For this review, take the finished solid that the model builds, in its own axes (mm). A direction names the side the tool comes from. Give positions to 0.01 mm unless a question says otherwise; leave off trailing zeros. Order: outer loops, then holes, each group sorted by start corner. A loop starts at its lowest first (then second) coordinate and runs counter-clockwise, first axis right, second up.
Item 1: For P1, Ø2, axis at x = -14.5, z = 5, coming from the -Y side; P2, Ø3, axis at x = -7, z = 9.5, coming from the -Y side; P3, Ø8, axis at x = -13.5, y = 2.5, coming from the +Z side, all flat-tipped, find the tip position at first contact; note any pin that passes through.
Item 2: Consider section D-D (y = 12). Give the boundary of the cut face in (x, z).
Item 3: For probe 1 along Z at (x, y) = (-6, -18); probe 2 along X at (y, z) = (-2, 17.25); probe 3 along X at (y, z) = (-0.5, 12.5), list the stretches that pass through material, from the lowest coordinate up.
Item 4: Machinability: for faces 1 (the cylindrical face through (-4.336, -19.524, 4.93)), 2 (the flat face through (4, -4, 10)), 3 (the cylindrical face through (0, -2, 2)), which of the approach directions +Z, -Z, +X, -X, +Y, -Y give a long, thin tool a straight path to every point of the face, cutting with its end or side? Answer none if there is none.
Item 5: Consider section B-B (x = 0). Give the boundary of the cut face in (y, z), plus the area to 3 significant figures.
Item 6: Consider section C-C (z = 6.5). Give the boundary of the cut face in (x, y), plus the area to 3 significant figures.
Item 7: The part is to be moulded in two halves that separate along Y. For faces 4 (the cylindrical face through (-1.08, -4.88, 16.41)), 5 (the flat face through (0, 0, 23)), 6 (the flat face through (0, 0, 5)), say which applies: released by +Y, released by -Y, zero draft, split by the parting line, or undercut.
Item 8: Consider section A-A (y = 0). Give the boundary of the cut face in (x, z), plus the area to 3 significant figures.
```python
from build123d import *

# Parameters (mm, degrees)
F0_R     = 20
F1_DEPTH = 10
F2_R     = 5
F3_DEPTH = 13
F5_DEPTH = 5


with BuildPart() as f1:
    # F0 (on Top) → F1 (new body)
    with BuildSketch(Plane.XY):
        Circle(F0_R)
    extrude(amount=F1_DEPTH)

    # F2 (on face) → F3 (join)
    with BuildSketch(Plane.XY.offset(10)):
        Circle(F2_R)
    extrude(amount=F3_DEPTH)

    # F4 (on face) → F5 (cut)
    with BuildSketch(Plane(origin=(0, 0, 0), x_dir=(1, 0, 0), z_dir=(0, 0, -1))):
        with BuildLine():
            Line((0, -1), (1.732051, -1))
            ThreePointArc((1.732051, -1), (0, 2), (-1.732051, -1))
            Line((-1.732051, -1), (0, -1))
        make_face()
    extrude(amount=-F5_DEPTH, mode=Mode.SUBTRACT)


solid = f1.part
```
Resolved:
1. P1: stops at y = -14.76
1. P2: stops at y = -19.23
1. P3: stops at z = 10
2. outline: (-16, 0) - (16, 0) - (16, 10) - (-16, 10) - close
3. probe 1: z = 0 to 10
3. probe 2: x = -4.58 to 4.58
3. probe 3: x = -4.97 to 4.97
4. face 1: +Z, -Z
4. face 2: +Z
4. face 3: -Z
5. outline: (-20, 0) - (-2, 0) - (-2, 5) - (1, 5) - (1, 0) - (20, 0) - (20, 10) - (5, 10) - (5, 23) - (-5, 23) - (-5, 10) - (-20, 10) - close
5. area: 515 mm2
6. outline: circle Ø40 at (0, 0)
6. area: 1,260 mm2
7. face 4: split by the parting line
7. face 5: zero draft
7. face 6: undercut
8. outline: (-20, 0) - (-2, 0) - (-2, 5) - (2, 5) - (2, 0) - (20, 0) - (20, 10) - (5, 10) - (5, 23) - (-5, 23) - (-5, 10) - (-20, 10) - close
8. area: 510 mm2
